```python
from build123d import *

# Parameters (mm, degrees)
SKETCH1_W                = 65
SKETCH1_H                = 15
BOSS_EXTRUDE1_DEPTH      = 7
SKETCH2_W                = 20.4
SKETCH2_H                = 15
CUT_EXTRUDE1_DEPTH       = 2
SKETCH3_R                = 1.7
CUT_EXTRUDE2_DEPTH       = 68.074585351
SKETCH4_R                = 3
CUT_EXTRUDE3_DEPTH       = 3.3
SKETCH5_R                = 2.2
CUT_EXTRUDE4_DEPTH       = 68.074585351
CHAMFER1_SIZE            = 1
BOSS_EXTRUDE2_DEPTH      = 5
BOSS_EXTRUDE2_DEPTH_BACK = 5
CUT_EXTRUDE5_DEPTH       = 69.600291545
CUT_EXTRUDE5_DEPTH_BACK  = 69.600291545
SKETCH7_W                = 9.39
SKETCH7_H                = 5.83
FILLET1_R                = 1.5
FILLET2_R                = 2
FILLET3_R                = 2
FILLET4_R                = 2
SKETCH8_R                = 1.25
CUT_EXTRUDE6_DEPTH       = 4.805
FILLET5_R                = 2


with BuildPart() as part:
    # Sketch1 → Boss-Extrude1 (new body)
    with BuildSketch(Plane(origin=(0, 0, 0), x_dir=(1, 0, 0), z_dir=(0, 1, 0))):
        with Locations((32.5, 7.5)):
            Rectangle(SKETCH1_W, SKETCH1_H)
    extrude(amount=BOSS_EXTRUDE1_DEPTH)

    # Sketch2 → Cut-Extrude1 (cut)
    with BuildSketch(Plane(origin=(0, 7, 0), x_dir=(1, 0, 0), z_dir=(0, 1, 0))):
        with Locations((32.5, 7.5)):
            Rectangle(SKETCH2_W, SKETCH2_H)
    extrude(amount=-CUT_EXTRUDE1_DEPTH, mode=Mode.SUBTRACT)

    # Sketch3 → Cut-Extrude2 (cut, through all)
    with BuildSketch(Plane(origin=(0, 0, 0), x_dir=(-1, 0, 0), z_dir=(0, -1, 0))):
        with Locations(Location((-32.5, 7.5, 0), (0, 0, 90))):
            Circle(SKETCH3_R)
    extrude(amount=-CUT_EXTRUDE2_DEPTH, mode=Mode.SUBTRACT)

    # Sketch4 → Cut-Extrude3 (cut)
    with BuildSketch(Plane(origin=(0, 0, 0), x_dir=(-1, 0, 0), z_dir=(0, -1, 0))):
        with Locations(Location((-32.5, 7.5, 0), (0, 0, 90))):
            Circle(SKETCH4_R)
    extrude(amount=-CUT_EXTRUDE3_DEPTH, mode=Mode.SUBTRACT)

    # Sketch5 → Cut-Extrude4 (cut, through all)
    with BuildSketch(Plane(origin=(0, 0, 0), x_dir=(-1, 0, 0), z_dir=(0, -1, 0))):
        with Locations(Location((-5.75, 7.5, 0), (0, 0, 90))):
            Circle(SKETCH5_R)
        with Locations(Location((-59.25, 7.5, 0), (0, 0, 90))):
            Circle(SKETCH5_R)
    extrude(amount=-CUT_EXTRUDE4_DEPTH, mode=Mode.SUBTRACT)

    # Chamfer1
    chamfer1_edges = [part.edges().sort_by_distance(p)[0] for p in [
        (5.75, 0, -5.3),
        (59.25, 0, -5.3),
    ]]
    chamfer(chamfer1_edges, length=CHAMFER1_SIZE)

    # Sketch6 → Boss-Extrude2 (add, two sides: drawn at the far end of the back side and taken through both)
    with BuildSketch(Plane.XY.offset(-1.658).offset(-BOSS_EXTRUDE2_DEPTH_BACK)):
        Polygon((-16.575, 22), (-16.575, 18.5), (-11.575, 18.5), (-11.575, 22), (0, 22), (0, 7), (0, 0), (-5, 0), (-5, 16), (-23.575, 16), (-23.575, 22), align=None)
    extrude(amount=BOSS_EXTRUDE2_DEPTH + BOSS_EXTRUDE2_DEPTH_BACK)

    # Sketch7 → Cut-Extrude5 (cut, two sides: drawn at the far end of the back side and taken through both)
    with BuildSketch(Plane.XZ.offset(-16).offset(-CUT_EXTRUDE5_DEPTH_BACK)):
        with Locations((-14.075, -1.658)):
            Rectangle(SKETCH7_W, SKETCH7_H)
    extrude(amount=CUT_EXTRUDE5_DEPTH + CUT_EXTRUDE5_DEPTH_BACK, mode=Mode.SUBTRACT)

    # Fillet1
    fillet1_edges = [part.edges().sort_by_distance(p)[0] for p in [
        (-16.575, 22, -5.6155),
        (-11.575, 22, -5.6155),
        (-23.575, 19, -6.658),
        (-23.575, 19, 3.342),
        (-11.575, 22, 2.2995),
        (-16.575, 22, 2.2995),
    ]]
    fillet(fillet1_edges, radius=FILLET1_R)

    # Fillet2
    fillet2_edges = [part.edges().sort_by_distance(p)[0] for p in [
        (-5, 0, -1.658),
        (-5, 16, -1.658),
    ]]
    fillet(fillet2_edges, radius=FILLET2_R)

    # Fillet3
    fillet3_edges = [part.edges().sort_by_distance(p)[0] for p in [
        (0, 22, -1.658),
    ]]
    fillet(fillet3_edges, radius=FILLET3_R)

    # Fillet4
    fillet4_edges = [part.edges().sort_by_distance(p)[0] for p in [
        (0, 3.5, -6.658),
        (0, 3.5, 0),
    ]]
    fillet(fillet4_edges, radius=FILLET4_R)

    # Sketch8 → Cut-Extrude6 (cut)
    with BuildSketch(Plane.ZY.offset(23.575)):
        with Locations((-1.508, 19)):
            Circle(SKETCH8_R)
    extrude(amount=-CUT_EXTRUDE6_DEPTH, mode=Mode.SUBTRACT)

    # Fillet5
    fillet5_edges = [part.edges().sort_by_distance(p)[0] for p in [
        (-1, 7, -6.658),
        (0, 7, -2.329),
    ]]
    fillet(fillet5_edges, radius=FILLET5_R - 0.0001)  # a hair under: the kernel refuses the full size


solid = part.part
```
Source: CAD feature listing. Evaluate the final solid. Frame: model axes, mm. A direction names the side the tool comes from. Coordinates: 2 decimals unless noted, no trailing zeros. Loops run counter-clockwise (first coordinate to the right, second up) from the corner with the lowest first, then second, coordinate; pieces in that order, holes last. Notation, with made-up numbers: M 69.25,-40 L 82.25,-40 A17 ccw 82.25,-11 Z; hole C 76.25,85.5 d8. An arc over 180 degrees is marked long. Use a Markdown table: item, result. Add a question column.
Q1. Material intervals for L1, parallel to X at y = 2.1, z = -7.5; L2, parallel to X at y = 3.25, z = -8.25; L3, parallel to Y at x = 11, z = -6.5, sorted ascending.
Q2. Section query A-A, the plane x = 32.5. Return loops of the section in (y, z).
Q3. Section query B-B, the plane y = 6. Return loops of the section in (x, z).
Q4. First-contact query: pin 1 (3 mm diameter, centred on y = 8.5, z = -4, fed in from -X); pin 2 (2 mm diameter, centred on y = 19, z = -1.508, fed in from +X); pin 3 (11 mm diameter, centred on x = -9.5, y = 6.5, fed in from -Z). Flat tips, straight axial feed; report the tip coordinate or a pass-through.
Q5. Section query C-C, the plane z = -7.5. State how many separate pieces and enclosed holes the cut face has, and give its area (3 significant figures).
Q6. Access query for faces 4 (the flat face through (0, 3, -12)), 5 (the flat face through (-19, 16, -2)), 6 (the flat face through (30, 5, -8)), 7 (the flat face through (-18.77, 19, -3)). Directions: +Z, -Z, +X, -X, +Y, -Y. A direction counts if a zero-diameter tool reaches every point of the face in a straight line with its end or side. Return the directions, or none.
Q7. Section query D-D, the plane x = 5.75. Return loops of the section in (y, z).
Q8. Draft query along Z for faces 1 (the flat face through (22.3, 6, -7)), 2 (the flat face through (32, 3, -15)), 3 (the cylindrical face through (7.605, 3.958, -8.683)). Return one class per face: pulls with the +Z half, pulls with the -Z half, needs draft (parallel to the pull), parting line crosses it, or undercut.
Result:
| question | item | result |
|---|---|---|
| 1 | L1 | x = -0.37 to 3.55, 7.95 to 29.5, 35.5 to 57.05, 61.45 to 65 |
| 1 | L2 | x = -0.04 to 3.68, 7.82 to 29.6, 35.4 to 57.18, 61.32 to 65 |
| 1 | L3 | y = 0 to 7 |
| 2 | outline | M 0,-15 L 5,-15 L 5,-9.2 L 3.3,-9.2 L 3.3,-10.5 L 0,-10.5 Z; M 0,-4.5 L 3.3,-4.5 L 3.3,-5.8 L 5,-5.8 L 5,0 L 0,0 Z |
| 3 | outline | M -5,-6.66 L -2,-6.66 A2 cw 0,-8.66 L 0,-15 L 22.3,-15 L 22.3,0 L 2,0 A2 cw 0,2 L 0,3.34 L -5,3.34 Z; M 42.7,-15 L 65,-15 L 65,0 L 42.7,0 Z; hole C 5.75,-7.5 d4.4; hole C 59.25,-7.5 d4.4 |
| 4 | pin 1 | stops at x = -5 |
| 4 | pin 2 | stops at x = 0 |
| 4 | pin 3 | stops at z = -6.66 |
| 5 | separate pieces | 4 |
| 5 | enclosed holes | 0 |
| 5 | area | 328 mm2 |
| 6 | face 4 | -Z, -X, +Y, -Y |
| 6 | face 5 | +Z, -Z, -X, -Y |
| 6 | face 6 | +Z, -Z, +Y |
| 6 | face 7 | +Y, -Y |
| 7 | outline | M 0,-15 L 7,-15 L 7,-9.7 L 1,-9.7 L 0,-10.7 Z; M 0,-4.3 L 1,-5.3 L 7,-5.3 L 7,0 L 0,0 Z |
| 8 | face 1 | needs draft |
| 8 | face 2 | pulls with the -Z half |
| 8 | face 3 | undercut |
